Autodesk Inventor part; units mm, degrees
ref_plane "YZ Plane" through (0, 0, 0) normal (1, 0, 0) x (0, 1, 0)
ref_plane "XZ Plane" through (0, 0, 0) normal (0, 1, 0) x (-1, 0, 0)
ref_plane "XY Plane" through (0, 0, 0) normal (0, 0, 1) x (1, 0, 0)
sketch "Sketch1" plane through (0, 0, 0) normal (0, 1, 0) x (-1, 0, 0)
  circle A0 centre (0, 0) radius 2.925
  line L0 (0, 10.1) -> (0, -10.1) construction
  arc A1 (1.9158, 10.2879) -> (-1.9158, 10.2879) centre (0, 10.1) ccw
  arc A2 (-1.9158, -10.2879) -> (1.9158, -10.2879) centre (0, -10.1) ccw
  line L1 (10.1, 0) -> (-10.1, 0) construction
  arc A3 (10.2879, -1.9158) -> (10.2879, 1.9158) centre (10.1, 0) ccw
  arc A4 (-10.2879, 1.9158) -> (-10.2879, -1.9158) centre (-10.1, 0) ccw
  line L2 (1.9158, 10.2879) -> (2.925, 0)
  line L3 (-1.9158, 10.2879) -> (-2.925, 0)
  line L4 (-2.925, 0) -> (-1.9158, -10.2879)
  line L5 (2.925, 0) -> (1.9158, -10.2879)
  line L6 (10.2879, 1.9158) -> (0, 2.925)
  line L7 (10.2879, -1.9158) -> (0, -2.925)
  line L8 (-10.2879, 1.9158) -> (0, 2.925)
  line L9 (-10.2879, -1.9158) -> (0, -2.925)
  point P0 (2.6637, 2.6637)
  point P1 (-2.6637, 2.6637)
  point P2 (-2.6637, -2.6637)
  point P3 (2.6637, -2.6637)
  point P4 (-0.5684, -2.8692)
  point P5 (0.5684, -2.8692)
  point P6 (2.8692, -0.5684)
  point P7 (2.8692, 0.5684)
  point P8 (0.5684, 2.8692)
  point P9 (-0.5684, 2.8692)
  point P10 (-2.8692, 0.5684)
  point P11 (-2.8692, -0.5684)
  dimension "d0" = 5.85
  dimension "d1" = 20.2
  dimension "d2" = 3.85
  dimension "d3" = 3.85
  dimension "d4" = 20.2
extrude "Extrusion1" add sketch "Sketch1" along normal blind 1.5 contours A0 L2 L6 A3 L7 L5 | A0 L6 L2 | L5 L7 A0 | A0 L8 L3 A1 L2 L6 | L7 L5 A2 L4 L9 A0 | A0 L3 L8 | L9 L4 A0 | A0 L4 L9 A4 L8 L3
extrude "Extrusion2" add sketch "Sketch1" along normal blind 2.2 and the other way blind 1.75 contours L5 A0 L7 L9 L4 L3 L8 L6 L2
sketch "Sketch2" plane through (0, -1.75, 0) normal (0, -1, 0) x (1, 0, 0)
  circle A0 centre (0, 0) radius 2.35
  dimension "d14" = 4.7
extrude "Extrusion3" cut sketch "Sketch2" against normal blind 2.95
sketch "Sketch3" plane through (0, 2.2, 0) normal (0, 1, 0) x (1, 0, 0)
  circle A0 centre (0, 0) radius 1
  dimension "d17" = 2
extrude "Extrusion4" cut sketch "Sketch3" against normal blind 2.95
sketch "Sketch4" plane through (0, 2.2, 0) normal (0, 1, 0) x (1, 0, 0)
  circle A0 centre (0, 0) radius 1
  circle A1 centre (0, 0) radius 2.35
  dimension "d20" = 4.7
extrude "Extrusion5" cut sketch "Sketch4" against normal blind 0.2 contours A0 | A1
properties part number "helice_cruz_mockup"
Input: part model. Units: mm. Frame: model coordinates. A direction names the side the tool comes from. Coordinates: 2 decimals unless noted, no trailing zeros. Order: outer loops, then holes, each group sorted by start corner. A loop starts at its lowest first (then second) coordinate and runs counter-clockwise, first axis right, second up. Notation, with made-up numbers: M -6,71 L 35,71 A31 cw 35,101 Z; hole C -29,-3 d4. An arc over 180 degrees is marked long. One line per question, with ' | ' between items.
Item 1: Section A-A (y = -0.85). Output: boundary loops of the cut face in (x, z) (3 decimals), then the cut area to 3 significant figures.
Geometry results:
outline: M -2.925,0 L -2.869,-0.568 A2.925 ccw -0.568,-2.869 L 0,-2.925 L 0.568,-2.869 A2.925 ccw 2.869,-0.568 L 2.925,0 L 2.869,0.568 A2.925 ccw 0.568,2.869 L 0,2.925 L -0.568,2.869 A2.925 ccw -2.869,0.568 Z; hole C 0,0 d4.7 | area: 9.49 mm^2
Item 2: Section C-C (x = 8). Output: boundary loops of the cut face in (y, z).
Geometry results:
outline: M 0,-2.14 L 1.5,-2.14 L 1.5,2.14 L 0,2.14 Z
Item 3: Reachability of faces 4 (the cylindrical face through (-2.051, -0.887, 2.085)), 5 (the cylindrical face through (2.085, -0.887, 2.051)), 6 (the flat face through (-3, 1.5, -2)) from +Z, -Z, +X, -X, +Y, -Y: full face, straight path, thin tool, end or side. Return the list, or none.
Geometry results:
face 4: +Z, -X, -Y | face 5: +Z, +X, -Y | face 6: +Y
Item 4: Pin query (flat end, axial travel): pin 1 (3 mm diameter, centred on x = -0.5, z = 0.5, fed in from +Y); pin 2 (8 mm diameter, centred on x = 8.5, z = 4.5, fed in from +Y); pin 3 (1.5 mm diameter, centred on x = 5, z = 3, fed in from -Y). Return the tip coordinate at first contact, or that it passes through.
Geometry results:
pin 1: stops at y = 2 | pin 2: stops at y = 1.5 | pin 3: stops at y = 0
Item 5: Ray query, line 1 along Z through (x, y) = (0, 2.15) (3 decimals); line 2 along Z through (x, y) = (0, 1.85) (3 decimals). Return the intervals inside material, ascending.
Geometry results:
line 1: z = -2.925 to -2.35, 2.35 to 2.925 | line 2: z = -2.925 to -1, 1 to 2.925
Item 6: Section D-D (z = 7). Output: boundary loops of the cut face in (x, y).
Geometry results:
outline: M -2.24,0 L 2.24,0 L 2.24,1.5 L -2.24,1.5 Z
Item 7: Draft query along Z for faces 1 (the flat face through (-2.285, 0.74, 6.529)), 2 (the cylindrical face through (2.051, -0.887, -2.085)), 3 (the cylindrical face through (-0.217, 1.606, 0.976)). Return one class per face: released by +Z, released by -Z, zero draft, split by the parting line, or undercut.
Geometry results:
face 1: released by +Z | face 2: released by -Z | face 3: undercut
